from build123d import *

# Parameters (mm, degrees)
SKETCH1_W           = 45
SKETCH1_H           = 20
BOSS_EXTRUDE1_DEPTH = 2.25
SKETCH2_W           = 2.25
SKETCH2_H           = 20
BOSS_EXTRUDE2_DEPTH = 10
SKETCH3_W           = 10
SKETCH3_H           = 20
BOSS_EXTRUDE3_DEPTH = 2.3
FILLET1_R           = 2
SKETCH4_R           = 2
CUT_EXTRUDE1_DEPTH  = 35.133927404
SKETCH5_R           = 2.5
BOSS_EXTRUDE4_DEPTH = 7
FILLET2_R           = 2
FILLET3_R           = 3


with BuildPart() as part:
    # Sketch1 → Boss-Extrude1 (new body)
    with BuildSketch(Plane(origin=(0, 0, 0), x_dir=(1, 0, 0), z_dir=(0, 1, 0))):
        Rectangle(SKETCH1_W, SKETCH1_H)
    extrude(amount=BOSS_EXTRUDE1_DEPTH)

    # Sketch2 → Boss-Extrude2 (add)
    with BuildSketch(Plane(origin=(0, 2.25, 0), x_dir=(1, 0, 0), z_dir=(0, 1, 0))):
        with Locations((-21.375, 0)):
            Rectangle(SKETCH2_W, SKETCH2_H)
        with Locations((21.375, 0)):
            Rectangle(SKETCH2_W, SKETCH2_H)
    extrude(amount=BOSS_EXTRUDE2_DEPTH)

    # Sketch3 → Boss-Extrude3 (add)
    with BuildSketch(Plane(origin=(0, 12.25, 0), x_dir=(1, 0, 0), z_dir=(0, 1, 0))):
        with Locations((-25.25, 0)):
            Rectangle(SKETCH3_W, SKETCH3_H)
        with Locations((25.25, 0)):
            Rectangle(SKETCH3_W, SKETCH3_H)
    extrude(amount=-BOSS_EXTRUDE3_DEPTH)

    # Fillet1
    fillet1_edges = [part.edges().sort_by_distance(p)[0] for p in [
        (-22.5, 9.95, 0),
        (22.5, 9.95, 0),
    ]]
    fillet(fillet1_edges, radius=FILLET1_R)

    # Sketch4 → Cut-Extrude1 (cut, through all)
    with BuildSketch(Plane(origin=(0, 12.25, 0), x_dir=(1, 0, 0), z_dir=(0, 1, 0))):
        with Locations(Location((26.45, 5.15278214, 0), (0, 0, 270))):
            Circle(SKETCH4_R)
        with Locations(Location((26.45, -5.15278214, 0), (0, 0, 270))):
            Circle(SKETCH4_R)
        with Locations(Location((-26.45, 5, 0), (0, 0, 270))):
            Circle(SKETCH4_R)
        with Locations(Location((-26.45, -5, 0), (0, 0, 270))):
            Circle(SKETCH4_R)
    extrude(amount=-CUT_EXTRUDE1_DEPTH, mode=Mode.SUBTRACT)

    # Sketch5 → Boss-Extrude4 (add)
    with BuildSketch(Plane.XZ):
        with Locations(Location((0, 0, 0), (0, 0, 270))):
            Circle(SKETCH5_R)
    extrude(amount=BOSS_EXTRUDE4_DEPTH)

    # Fillet2
    fillet2_edges = [part.edges().sort_by_distance(p)[0] for p in [
        (0, 0, 2.5),
    ]]
    fillet(fillet2_edges, radius=FILLET2_R)

    # Fillet3
    fillet3_edges = [part.edges().sort_by_distance(p)[0] for p in [
        (-30.25, 11.1, -10),
        (-30.25, 11.1, 10),
        (30.25, 11.1, 10),
        (30.25, 11.1, -10),
    ]]
    fillet(fillet3_edges, radius=FILLET3_R)


solid = part.part
Can you work these out from the model? Positions are in its coordinate system, mm. A direction names the side the tool comes from. Coordinates: 2 decimals unless noted, no trailing zeros. Loops run counter-clockwise (first coordinate to the right, second up) from the corner with the lowest first, then second, coordinate; pieces in that order, holes last. Notation, with made-up numbers: M 4,7.5 L 11,7.5 A28 ccw 11,37.5 Z; hole C 84.5,-33.5 d6. An arc over 180 degrees is marked long. Answer as CSV lines item,"result". Start each with the question number.
1. Suppose I cut it at B-B, the plane x = 26.45. List the corners of the cut face in (y, z) for me, plus the area to 3 significant figures.
2. Suppose I cut it at C-C, the plane z = 0. List the corners of the cut face in (x, y) for me.
3. Suppose I cut it at A-A, the plane y = 5.5. List the corners of the cut face in (x, z) for me, plus the area to 3 significant figures.
4. For pin 1 Ø1.5 at (x, y) = (-18, 10.5) entering from +Z; pin 2 Ø6.5 at (y, z) = (4.5, -0.5) entering from +X; pin 3 Ø3 at (x, z) = (14.5, 4) entering from -Y; pin 4 Ø3 at (x, z) = (-3.5, -4.5) entering from +Y, each with a flat end and sliding along its axis, tell me the tip position at first contact or that it passes through.
5. Thinking about a two-plate mould opening in Z: for faces 1 (the face through (-23.1, 9.38, -0.14)), 2 (the face through (-24.467, 11.116, -5.26)), 3 (the face through (24.5, 11.1, -5.6)), 4 (the face through (-29.35, 11.08, -9.14)), which applies, +Z half, -Z half, draft (parallel to the pull), parting line (faces both ways), or undercut?
6. If I drill on probe 1 along Z at (x, y) = (26.45, 11); probe 2 along Z at (x, y) = (-26.45, 11.25); probe 3 along X at (y, z) = (11.1, 5), over which ranges is the centre line in solid material (lowest first)? Write a range as [from, to].
7. Suppose I cut it at D-D, the plane y = -5. List the corners of the cut face in (x, z) for me.
8. For faces 5 (the face through (20.25, 7, 0)), 6 (the face through (0, -7, 0)), 7 (the face through (-2.44, -4.46, 0.54)), 8 (the face through (-22.5, 4, 0)), 9 (the face through (23.07, 9.35, -0.14)), which set-ups out of +Z, -Z, +X, -X, +Y, -Y let a thin tool reach every point of the face, with its end or its side?
Output:
1,outline,"M 9.95,-10 L 12.25,-10 L 12.25,-7.15 L 9.95,-7.15 Z; M 9.95,-3.15 L 12.25,-3.15 L 12.25,3.15 L 9.95,3.15 Z; M 9.95,7.15 L 12.25,7.15 L 12.25,10 L 9.95,10 Z"
1,area,"27.6 mm^2"
2,outline,"M -30.25,9.95 L -24.5,9.95 A2 cw -22.5,7.95 L -22.5,0 L -4.5,0 A2 cw -2.5,-2 L -2.5,-7 L 2.5,-7 L 2.5,-2 A2 cw 4.5,0 L 22.5,0 L 22.5,7.95 A2 cw 24.5,9.95 L 30.25,9.95 L 30.25,12.25 L 20.25,12.25 L 20.25,2.25 L -20.25,2.25 L -20.25,12.25 L -30.25,12.25 Z"
3,outline,"M -22.5,-10 L -20.25,-10 L -20.25,10 L -22.5,10 Z; M 20.25,-10 L 22.5,-10 L 22.5,10 L 20.25,10 Z"
3,area,"90.0 mm^2"
4,pin 1,"passes through"
4,pin 2,"stops at x = 22.5"
4,pin 3,"stops at y = 0"
4,pin 4,"stops at y = 2.25"
5,face 1,"draft"
5,face 2,"undercut"
5,face 3,"undercut"
5,face 4,"-Z half"
6,probe 1,"z = [-10, -7.15], [-3.15, 3.15], [7.15, 10]"
6,probe 2,"z = [-10, -7], [-3, 3], [7, 10]"
6,probe 3,"x = [-30.25, -28.45], [-24.45, -20.25], [20.25, 24.46], [28.44, 30.25]"
7,outline,"C 0,0 d5"
8,face 5,"+Z, -Z, +Y"
8,face 6,"+Z, -Z, +X, -X, -Y"
8,face 7,"-Y"
8,face 8,"+Z, -Z, -X, -Y"
8,face 9,"+Z, -Z, +X, -Y"
